Autodesk Inventor part; units mm, degrees
ref_plane "YZ Plane" through (0, 0, 0) normal (1, 0, 0) x (0, 1, 0)
ref_plane "XZ Plane" through (0, 0, 0) normal (0, 1, 0) x (-1, 0, 0)
ref_plane "XY Plane" through (0, 0, 0) normal (0, 0, 1) x (1, 0, 0)
sketch "スケッチ1" plane through (0, 0, 0) normal (0, 0, 1) x (1, 0, 0)
  line L0 (-5, -100) -> (5, -100)
  line L1 (5, -100) -> (5, 100)
  line L2 (5, 100) -> (-5, 100)
  line L3 (-5, 100) -> (-5, -100)
  line L4 (-5, -100) -> (5, 100) construction
  line L5 (5, -100) -> (-5, 100) construction
  point P0 (0, 0)
  dimension "d0" = 10
  dimension "d1" = 200
extrude "押し出し1" add sketch "スケッチ1" along normal blind 2
sketch "スケッチ2" plane through (0, 0, 2) normal (0, 0, 1) x (1, 0, 0)
  line L0 (5, 100) -> (-5, 100)
  point P0 (0, 0)
  point P1 (0, 100)
  point P2 (0, 90)
  point P3 (0, 70)
  dimension "d4" = 10
  dimension "d5" = 20
hole "穴1" at (0, 90, 2) at (0, 70, 2) direction (0, 0, -1) diameter 3.4 end through all
sketch "スケッチ3" plane through (0, 0, 0) normal (0, 0, -1) x (-1, 0, 0)
  line L0 (5, -100) -> (-5, -100)
  line L1 (-5, -100) -> (5, -100)
  line L2 (5, -100) -> (5, -98)
  line L3 (5, -98) -> (-5, -98)
  line L4 (-5, -98) -> (-5, -100)
  point P0 (0, 0)
  dimension "d13" = 2
extrude "押し出し2" add sketch "スケッチ3" along normal blind 20
sketch "スケッチ4" plane through (-5, -98, 0) normal (0, 1, 0) x (1, 0, 0)
  line L0 (0, 20) -> (10, 20)
  point P0 (5, 0)
  point P1 (5, 15)
  point P2 (5, 5)
  dimension "d16" = 5
  dimension "d17" = 10
hole "穴2" at (0, -98, -15) at (0, -98, -5) direction (0, -1, 0) diameter 3.4 end through all
properties part number "20220509_知能ロボットカメラ角棒"
CAD build for the part. Positions are in the model's coordinates, mm. Give positions to 0.01 mm unless a question says otherwise; leave off trailing zeros. Write each loop counter-clockwise with the first axis right and the second up, starting at its lowest first coordinate (ties: lowest second). Pieces come first, ordered by that corner, then holes. Notation, with made-up numbers: (40.5, -34) -> (67.5, -34) arc R19 cw to (67.5, -5) -> close; hole circle Ø3 at (77.5, 49.25). An arc over 180 degrees is marked (long way). Write each question's results on one line, items separated by ' | '.
1. Cut at B-B, the plane x = 0. Write the cut outline in (y, z), then the cut area to 3 significant figures.
Geometry check:
outline: (-100, -20) -> (-98, -20) -> (-98, -16.7) -> (-100, -16.7) -> close; (-100, -13.3) -> (-98, -13.3) -> (-98, -6.7) -> (-100, -6.7) -> close; (-100, -3.3) -> (-98, -3.3) -> (-98, 0) -> (68.3, 0) -> (68.3, 2) -> (-100, 2) -> close; (71.7, 0) -> (88.3, 0) -> (88.3, 2) -> (71.7, 2) -> close; (91.7, 0) -> (100, 0) -> (100, 2) -> (91.7, 2) -> close | area: 413 mm²
2. Wall check: probe 1 along Y at (x, z) = (0, 1.55); probe 2 along Z at (x, y) = (0, -99); probe 3 along X at (y, z) = (70, 0.5). Give the ranges that are in metal, low to high. Write a range as [from, to].
Geometry check:
probe 1: [-100, 68.3], [71.7, 88.3], [91.7, 100] | probe 2: [-20, -16.7], [-13.3, -6.7], [-3.3, 2] | probe 3: [-5, -1.7], [1.7, 5]
3. Cut at C-C, the plane z = -5. Write the cut outline in (x, y).
Geometry check:
outline: (-5, -100) -> (-1.7, -100) -> (-1.7, -98) -> (-5, -98) -> close; (1.7, -100) -> (5, -100) -> (5, -98) -> (1.7, -98) -> close
4. Two-plate mould, pull along Z, no slides. Class faces 1 (the flat face through (0, 2, 0)), 2 (the flat face through (0, -98, -10)), 3 (the cylindrical face through (-0.51, -99.01, -13.38)): pulls with the +Z half, pulls with the -Z half, needs draft (parallel to the pull), parting line crosses it, or undercut.
Geometry check:
face 1: pulls with the -Z half | face 2: needs draft | face 3: undercut
5. Drop flat-ended pins along their axis: P1, Ø3, axis at x = 0, y = 70, coming from the +Z side; P2, Ø1, axis at x = 3.5, y = -76, coming from the -Z side; P3, Ø5.5, axis at x = 0, z = -15, coming from the +Y side. Give the stop position or say it passes through.
Geometry check:
P1: through | P2: z = 0 | P3: y = -98
6. Cut at A-A, the plane y = 90. Write the cut outline in (x, z), then the cut area to 3 significant figures.
Geometry check:
outline: (-5, 0) -> (-1.7, 0) -> (-1.7, 2) -> (-5, 2) -> close; (1.7, 0) -> (5, 0) -> (5, 2) -> (1.7, 2) -> close | area: 13.2 mm²
7. Cut at D-D, the plane y = 59. Write the cut outline in (x, z), then the cut area to 3 significant figures.
Geometry check:
outline: (-5, 0) -> (5, 0) -> (5, 2) -> (-5, 2) -> close | area: 20.0 mm²
